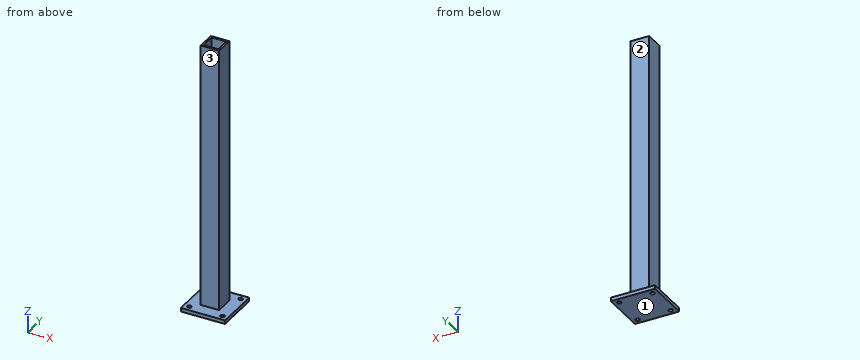
from build123d import *

# Parameters (mm, degrees)
F0_W     = 63.5
F0_H     = 914.4
F1_DEPTH = 63.5
F2_W     = 50.8
F2_H     = 50.8
F3_DEPTH = 914.401
F5_DEPTH = 12.7
F7_DEPTH = 25.4


with BuildPart() as f1:
    # F0 (on Front) → F1 (new body)
    with BuildSketch(Plane.XZ):
        with Locations((-31.75, 457.2)):
            Rectangle(F0_W, F0_H)
    extrude(amount=F1_DEPTH)

    # F2 (on face) → F3 (cut, through all)
    with BuildSketch(Plane(origin=(0, 0, 0), x_dir=(1, 0, 0), z_dir=(0, 0, -1))):
        with Locations((-31.75, 31.75)):
            Rectangle(F2_W, F2_H)
    extrude(amount=-F3_DEPTH, mode=Mode.SUBTRACT)

    # F4 (on face) → F5 (join)
    with BuildSketch(Plane(origin=(0, 0, 0), x_dir=(1, 0, 0), z_dir=(0, 0, -1))):
        Polygon((44.45, 107.95), (-63.5, 107.95), (-107.95, 107.95), (-107.95, -44.45), (44.45, -44.45), align=None)
    extrude(amount=F5_DEPTH)

    # F6 (on face) → F7 (cut)
    with BuildSketch(Plane.XY):
        with BuildLine():
            ThreePointArc((-81.75625, 25.4), (-88.9, 32.54375), (-96.04375, 25.4))
            Line((-96.04375, 25.4), (-81.75625, 25.4))
        make_face()
        with BuildLine():
            ThreePointArc((32.54375, 25.4), (25.4, 32.54375), (18.25625, 25.4))
            ThreePointArc((18.25625, 25.4), (25.4, 18.25625), (32.54375, 25.4))
        make_face()
        with BuildLine():
            Line((-81.75625, 25.4), (-96.04375, 25.4))
            ThreePointArc((-96.04375, 25.4), (-88.9, 18.25625), (-81.75625, 25.4))
        make_face()
        with BuildLine():
            ThreePointArc((-81.75625, -88.9), (-88.9, -81.75625), (-96.04375, -88.9))
            Line((-96.04375, -88.9), (-81.75625, -88.9))
        make_face()
        with BuildLine():
            ThreePointArc((32.54375, -88.9), (25.4, -81.75625), (18.25625, -88.9))
            Line((18.25625, -88.9), (32.54375, -88.9))
        make_face()
        with BuildLine():
            Line((32.54375, -88.9), (18.25625, -88.9))
            ThreePointArc((18.25625, -88.9), (25.4, -96.04375), (32.54375, -88.9))
        make_face()
        with BuildLine():
            Line((-81.75625, -88.9), (-96.04375, -88.9))
            ThreePointArc((-96.04375, -88.9), (-88.9, -96.04375), (-81.75625, -88.9))
        make_face()
    extrude(amount=-F7_DEPTH, mode=Mode.SUBTRACT)


solid = f1.part
Verification items for the finished model (mm, model axes). Face numbers are marked on the shaded views. A direction names the side the tool comes from. Round coordinates to 2 decimals unless told otherwise and drop trailing zeros. Loops run counter-clockwise (first coordinate to the right, second up) from the corner with the lowest first, then second, coordinate; pieces in that order, holes last. Notation, with made-up numbers: (70, -32) - (111, -32) arc R25 cw to (111, 5) - close; hole circle Ø5 at (58.25, 4). An arc over 180 degrees is marked (long way). Answer in a Markdown table with one row per item. Add a question column.
Q1. Section check B-B on y = -34. Enter the section's corners in (x, z).
Q2. Tool access check on the marked faces 1, 2 and 3. Record the directions out of +Z, -Z, +X, -X, +Y, -Y that give a thin tool (end or side, any length) a straight path to the whole face; none if there is none.
Q3. Material ranges on line 1 (Y direction, x = -88, z = -2); line 2 (X direction, y = 25.4, z = -3); line 3 (Y direction, x = -23, z = 524.5), recorded low to high.
Q4. Gauge pin test, flat ends, axial feed: pin 1 (12 mm diameter, centred on x = 4.5, z = 280.5, fed in from -Y); pin 2 (13 mm diameter, centred on x = 25.4, y = -88.9, fed in from +Z); pin 3 (16.5 mm diameter, centred on x = -88.9, y = -88.9, fed in from -Z); pin 4 (18.5 mm diameter, centred on x = -88.9, y = 25.4, fed in from +Z). Record the tip position at first contact, or that the pin passes through.
Q5. Section check A-A on z = 532. Enter the section's corners in (x, y), plus the area to 3 significant figures.
Found:
| question | item | result |
|---|---|---|
| 1 | outline | (-107.95, -12.7) - (44.45, -12.7) - (44.45, 0) - (0, 0) - (0, 914.4) - (-6.35, 914.4) - (-6.35, 0) - (-57.15, 0) - (-57.15, 914.4) - (-63.5, 914.4) - (-63.5, 0) - (-107.95, 0) - close |
| 2 | face 1 | -Z, +X, -X, +Y, -Y |
| 2 | face 2 | +Z, +X, -X, +Y |
| 2 | face 3 | +Z, +X, -X, -Y |
| 3 | line 1 | y = -107.95 to -95.99, -81.81 to 18.31, 32.49 to 44.45 |
| 3 | line 2 | x = -107.95 to -96.04, -81.76 to 18.26, 32.54 to 44.45 |
| 3 | line 3 | y = -63.5 to -57.15, -6.35 to 0 |
| 4 | pin 1 | stops at y = -63.5 |
| 4 | pin 2 | passes through |
| 4 | pin 3 | stops at z = -12.7 |
| 4 | pin 4 | stops at z = 0 |
| 5 | outline | (-63.5, -63.5) - (0, -63.5) - (0, 0) - (-63.5, 0) - close; hole (-57.15, -57.15) - (-6.35, -57.15) - (-6.35, -6.35) - (-57.15, -6.35) - close |
| 5 | area | 1,450 mm² |
